Verification items for the finished model (mm, model axes). Face numbers are marked on the shaded views. A direction names the side the tool comes from. Round coordinates to 2 decimals unless told otherwise and drop trailing zeros. Write each loop counter-clockwise with the first axis right and the second up, starting at its lowest first coordinate (ties: lowest second). Pieces come first, ordered by that corner, then holes. Notation, with made-up numbers: (10, 80.5) - (39, 80.5) arc R25 ccw to (39, 92.5) - close; hole circle Ø7 at (-26, 14.25). An arc over 180 degrees is marked (long way). Answer as a JSON object with one key per item and string values. Group by question number.
1) Set-up check for the marked faces 1, 2 and 3: record each of +Z, -Z, +X, -X, +Y, -Y from which the full face is reachable in a straight line by a thin tool's end or side.
2) Section check A-A (y = 0). Enter the section's corners in (x, z).
3) Thickness scan on line 1 (X direction, y = 9.5, z = 255); line 2 (Y direction, x = 18, z = 263.5); line 3 (Z direction, x = -9.5, y = -19.5). Record the ranges inside material, lowest first.
4) Section check D-D (z = 260). Enter the section's corners in (x, y).
5) Section check C-C (x = 19.5). Enter the section's corners in (y, z), then the cut area to 3 significant figures.
6) Mould release check, pull along Y, two halves, no side actions. Record for the marked faces 4, 5 and 6: +Y half, -Y half, draft (parallel to the pull), parting line (faces both ways), or undercut.
7) Go/stop test with flat-tipped pins: pin 1 Ø5 at (x, z) = (2, 259) entering from -Y; pin 2 Ø1.8 at (y, z) = (9.5, 240) entering from +X; pin 3 Ø0.8 at (x, y) = (-1.5, 12.5) entering from -Z; pin 4 Ø5 at (x, y) = (-14.27, 8) entering from -Z. Record where each tip stops, or that it passes through.
8) Section check B-B (z = 252.5). Enter the section's corners in (x, y), then the cut area to 3 significant figures.
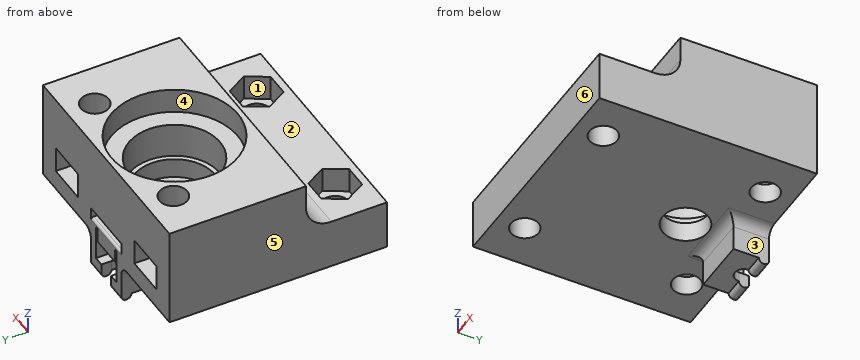
```python
from build123d import *

# Parameters (mm, degrees)
BOSS_EXTRUDE1_DEPTH      = 13.5
BOSS_EXTRUDE2_DEPTH      = 18.5
BOSS_EXTRUDE3_DEPTH      = 5
SKETCH4_W                = 45.922011884
SKETCH4_H                = 20
BOSS_EXTRUDE4_DEPTH      = 13.5
SKETCH2_R                = 4.25
CUT_EXTRUDE1_DEPTH       = 268.629329099
SKETCH6_R                = 9
CUT_EXTRUDE3_DEPTH       = 12
SKETCH7_R                = 12.5
CUT_EXTRUDE4_DEPTH       = 5
BOSS_EXTRUDE5_DEPTH      = 13.5
CUT_EXTRUDE5_REACH       = 210.1
CUT_EXTRUDE5_END_RADIUS  = 45
SKETCH8_R                = 9
CUT_EXTRUDE6_REACH       = 210.1
SKETCH10_R               = 4
SKETCH11_R               = 8
CUT_EXTRUDE7_DEPTH       = 4
SKETCH18_R               = 11
CUT_EXTRUDE9_DEPTH       = 47
CUT_EXTRUDE11_DEPTH      = 268.629329099
CUT_EXTRUDE11_DEPTH_BACK = 268.629329099
SKETCH20_W               = 45.922011884
SKETCH20_H               = 204.425421037
SKETCH21_W               = 45.922011884
SKETCH21_H               = 10
BOSS_EXTRUDE6_DEPTH      = 16
M5_CLEARANCE_HOLE1_D     = 5.5
CUT_EXTRUDE12_DEPTH      = 5
FILLET1_R                = 5
LPATTERN2_COUNT          = 2
LPATTERN2_PITCH          = 32
LPATTERN2_COPY_1_D       = 5.5
CUT_EXTRUDE13_START      = -9.2
SKETCH25_R               = 2.75
CUT_EXTRUDE13_DEPTH      = 5.2
SKETCH26_R               = 8.05
CUT_EXTRUDE14_DEPTH      = 4
SKETCH27_W               = 11
SKETCH27_H               = 7
BOSS_EXTRUDE7_DEPTH      = 5
CUT_EXTRUDE15_DEPTH      = 5
FILLET2_R                = 2
BOSS_EXTRUDE8_DEPTH      = 2
BOSS_EXTRUDE9_DEPTH      = 3.75
SKETCH31_W               = 11
SKETCH31_H               = 2.1
CUT_EXTRUDE16_DEPTH      = 2.5
FILLET3_R                = 0.5
CUT_EXTRUDE17_REACH      = 44.396
SKETCH32_R               = 4.5


with BuildPart() as part:
    # Sketch1 → Boss-Extrude1 (new, symmetric)
    with BuildSketch(Plane(origin=(0, 0, 0), x_dir=(1, 0, 0), z_dir=(0, 1, 0))):
        with BuildLine():
            ThreePointArc((17.220754456, -41.574578963), (0, -45), (-17.220754456, -41.574578963))
            Line((-17.220754456, -41.574578963), (-22.961005942, -55.432771951))
            ThreePointArc((-22.961005942, -55.432771951), (0, -60), (22.961005942, -55.432771951))
            Line((22.961005942, -55.432771951), (17.220754456, -41.574578963))
        make_face()
    extrude(amount=BOSS_EXTRUDE1_DEPTH, both=True)

    # Sketch1_3 → Boss-Extrude2 (add, symmetric)
    with BuildSketch(Plane(origin=(0, 0, 0), x_dir=(1, 0, 0), z_dir=(0, 1, 0))):
        with BuildLine():
            ThreePointArc((19.134171618, -46.193976626), (0, -50), (-19.134171618, -46.193976626))
            Line((-19.134171618, -46.193976626), (-21.04758878, -50.813374288))
            ThreePointArc((-21.04758878, -50.813374288), (0, -55), (21.04758878, -50.813374288))
            Line((21.04758878, -50.813374288), (19.134171618, -46.193976626))
        make_face()
    extrude(amount=BOSS_EXTRUDE2_DEPTH, both=True)

    # Sketch3 → Boss-Extrude3 (add, symmetric)
    with BuildSketch(Plane.XZ):
        with BuildLine():
            Line((-22.961005942, 266), (-22.961005942, 55.432771951))
            ThreePointArc((-22.961005942, 55.432771951), (-20.481139434, 56.39612511), (-17.961005942, 57.248600555))
            Line((-17.961005942, 57.248600555), (-17.961005942, 246))
            Line((-17.961005942, 246), (17.961005942, 246))
            Line((17.961005942, 246), (17.961005942, 57.248600555))
            ThreePointArc((17.961005942, 57.248600555), (20.481139434, 56.39612511), (22.961005942, 55.432771951))
            Line((22.961005942, 55.432771951), (22.961005942, 266))
            Line((22.961005942, 266), (-22.961005942, 266))
        make_face()
    extrude(amount=BOSS_EXTRUDE3_DEPTH, both=True)

    # Sketch4 → Boss-Extrude4 (add, symmetric)
    with BuildSketch(Plane(origin=(0, 0, 0), x_dir=(1, 0, 0), z_dir=(0, 1, 0))):
        with Locations((0, -256)):
            Rectangle(SKETCH4_W, SKETCH4_H)
    extrude(amount=BOSS_EXTRUDE4_DEPTH, both=True)

    # Sketch2 → Cut-Extrude1 (cut, through all)
    with BuildSketch(Plane.XY):
        with Locations(Location((0, 0, 0), (0, 0, 180))):
            Circle(SKETCH2_R)
    extrude(amount=CUT_EXTRUDE1_DEPTH, mode=Mode.SUBTRACT)

    # Sketch6 → Cut-Extrude3 (cut)
    with BuildSketch(Plane.XY.offset(266)):
        Circle(SKETCH6_R)
    extrude(amount=-CUT_EXTRUDE3_DEPTH, mode=Mode.SUBTRACT)

    # Sketch7 → Cut-Extrude4 (cut)
    with BuildSketch(Plane.XY.offset(266)):
        Circle(SKETCH7_R)
    extrude(amount=-CUT_EXTRUDE4_DEPTH, mode=Mode.SUBTRACT)

    # Sketch9 → Boss-Extrude5 (add, symmetric)
    with BuildSketch(Plane(origin=(0, 0, 0), x_dir=(1, 0, 0), z_dir=(0, 1, 0))):
        with BuildLine():
            Line((-22.961005942, -55.432771951), (-22.961005942, -68))
            Line((-22.961005942, -68), (22.961005942, -68))
            Line((22.961005942, -68), (22.961005942, -55.432771951))
            ThreePointArc((22.961005942, -55.432771951), (0, -60), (-22.961005942, -55.432771951))
        make_face()
    extrude(amount=BOSS_EXTRUDE5_DEPTH, both=True)

    # Cut-Extrude5: up to this cylinder (the profile starts outside it)
    cut_extrude5_end = Plane(origin=(0, 0, 0), z_dir=(0, -1, 0)) * Cylinder(CUT_EXTRUDE5_END_RADIUS, 511.2, mode=Mode.PRIVATE)
    # Sketch8 → Cut-Extrude5 (cut, up to the surface)
    with BuildSketch(Plane.XY.offset(60), mode=Mode.PRIVATE) as cut_extrude5_sk1:
        Circle(SKETCH8_R)
    cut_extrude5_tool1 = extrude(cut_extrude5_sk1.sketch, amount=-CUT_EXTRUDE5_REACH, mode=Mode.PRIVATE) - cut_extrude5_end
    add(cut_extrude5_tool1.solids().sort_by_distance((0, 0, 60))[0], mode=Mode.SUBTRACT)

    # Sketch10 → Cut-Extrude6 (cut, up to next)
    with BuildSketch(Plane.XY.offset(60), mode=Mode.PRIVATE) as cut_extrude6_sk1:
        with Locations(Location((0, 0, 0), (0, 0, 180))):
            Circle(SKETCH10_R)
    cut_extrude6_tool1 = extrude(cut_extrude6_sk1.sketch, amount=CUT_EXTRUDE6_REACH, mode=Mode.PRIVATE) & part.part
    add(cut_extrude6_tool1.solids().sort_by_distance((0, 0, 60))[0], mode=Mode.SUBTRACT)

    # Sketch11 → Cut-Extrude7 (cut)
    with BuildSketch(Plane.XY.offset(68)):
        Circle(SKETCH11_R)
    extrude(amount=-CUT_EXTRUDE7_DEPTH, mode=Mode.SUBTRACT)

    # Sketch18 → Cut-Extrude9 (cut)
    with BuildSketch(Plane.XY):
        with Locations(Location((0, 0, 0), (0, 0, 180))):
            Circle(SKETCH18_R)
    extrude(amount=CUT_EXTRUDE9_DEPTH, mode=Mode.SUBTRACT)

    # Sketch20 → Cut-Extrude11 (cut, two sides: drawn at the far end of the back side and taken through both)
    with BuildSketch(Plane(origin=(0, 0, 0), x_dir=(1, 0, 0), z_dir=(0, 1, 0)).offset(-CUT_EXTRUDE11_DEPTH_BACK)):
        with Locations((0, -143.787289482)):
            Rectangle(SKETCH20_W, SKETCH20_H)
    extrude(amount=CUT_EXTRUDE11_DEPTH + CUT_EXTRUDE11_DEPTH_BACK, mode=Mode.SUBTRACT)

    # Sketch21 → Boss-Extrude6 (add)
    with BuildSketch(Plane.XZ.offset(13.5)):
        with Locations((0, 251)):
            Rectangle(SKETCH21_W, SKETCH21_H)
    extrude(amount=BOSS_EXTRUDE6_DEPTH)

    # M5 Clearance Hole1 (through all)
    with Locations(Plane(origin=(0, 0, 246), x_dir=(-1, 0, 0), z_dir=(0, 0, -1))):
        with Locations((-14.26606865, -24)):
            m5_clearance_hole1 = Hole(M5_CLEARANCE_HOLE1_D / 2)

    # Sketch24 → Cut-Extrude12 (cut)
    with BuildSketch(Plane.XY.offset(256)):
        Polygon((18.94260583, -24), (16.60433724, -19.95), (11.92780006, -19.95), (9.58953147, -24), (11.92780006, -28.05), (16.60433724, -28.05), align=None)
    cut_extrude12 = extrude(amount=-CUT_EXTRUDE12_DEPTH, mode=Mode.SUBTRACT)

    # Mirror1: M5 Clearance Hole1 across plane
    add(m5_clearance_hole1.mirror(Plane(origin=(0, 0, 0), x_dir=(0, 0, 1), z_dir=(1, 0, 0))), mode=Mode.SUBTRACT)

    # Mirror2: Cut-Extrude12 across plane
    add(cut_extrude12.mirror(Plane(origin=(0, 0, 0), x_dir=(0, 0, 1), z_dir=(1, 0, 0))), mode=Mode.SUBTRACT)

    # Fillet1
    fillet1_edges = [part.edges().sort_by_distance(p)[0] for p in [
        (0, -13.5, 256),
    ]]
    fillet(fillet1_edges, radius=FILLET1_R)

    # LPattern2: M5 Clearance Hole1 ×2
    with Locations(*[(0, i * LPATTERN2_PITCH, 0) for i in range(1, LPATTERN2_COUNT)]):
        add(m5_clearance_hole1, mode=Mode.SUBTRACT)

    # LPattern2 copy 1 (through all)
    with Locations(Plane(origin=(0, 32, 246), x_dir=(1, 0, 0), z_dir=(0, 0, -1))):
        with Locations((-14.26606865, 24)):
            Hole(LPATTERN2_COPY_1_D / 2)

    # Sketch25 → Cut-Extrude13 (cut)
    # profile 1 of 2: a face of its own
    with BuildSketch(Plane(origin=(0, 0, 246), x_dir=(-1, 0, 0), z_dir=(0, 0, -1)).offset(CUT_EXTRUDE13_START)):
        Polygon((-18.31606865, 13.5), (-18.31606865, 10.33826859), (-14.26606865, 12.67653718), (-10.21606865, 10.33826859), (-10.21606865, 13.5), align=None)
    # profile 2 of 2: a face of its own
    with BuildSketch(Plane(origin=(0, 0, 246), x_dir=(-1, 0, 0), z_dir=(0, 0, -1)).offset(CUT_EXTRUDE13_START)):
        Polygon((-10.21606865, 10.33826859), (-14.26606865, 12.67653718), (-18.31606865, 10.33826859), (-18.31606865, 5.66173141), (-14.26606865, 3.32346282), (-10.21606865, 5.66173141), align=None)
        with Locations((-14.26606865, 8)):
            Circle(SKETCH25_R, mode=Mode.SUBTRACT)
    cut_extrude13 = extrude(amount=CUT_EXTRUDE13_DEPTH, mode=Mode.SUBTRACT)

    # Mirror3: Cut-Extrude13 across plane
    add(cut_extrude13.mirror(Plane(origin=(0, 0, 0), x_dir=(0, 0, 1), z_dir=(1, 0, 0))), mode=Mode.SUBTRACT)

    # Sketch26 → Cut-Extrude14 (cut)
    with BuildSketch(Plane.XY.offset(254)):
        Circle(SKETCH26_R)
    extrude(amount=-CUT_EXTRUDE14_DEPTH, mode=Mode.SUBTRACT)

    # Sketch27 → Boss-Extrude7 (add)
    with BuildSketch(Plane(origin=(0, 0, 246), x_dir=(-1, 0, 0), z_dir=(0, 0, -1))):
        with Locations((0, 10)):
            Rectangle(SKETCH27_W, SKETCH27_H)
    extrude(amount=BOSS_EXTRUDE7_DEPTH)

    # Sketch28 → Cut-Extrude15 (cut)
    with BuildSketch(Plane(origin=(0, 13.5, 0), x_dir=(1, 0, 0), z_dir=(0, 1, 0))):
        Polygon((-3.735, -241), (3.735, -241), (3.735, -248), (3.235, -248), (3.235, -245.2), (-3.235, -245.2), (-3.235, -248), (-3.735, -248), align=None)
    extrude(amount=-CUT_EXTRUDE15_DEPTH, mode=Mode.SUBTRACT)

    # Fillet2
    fillet2_edges = [part.edges().sort_by_distance(p)[0] for p in [
        (5.5, 10, 246),
        (0, 6.5, 246),
        (-5.5, 10, 246),
    ]]
    fillet(fillet2_edges, radius=FILLET2_R)

    # Sketch29 → Boss-Extrude8 (add)
    with BuildSketch(Plane(origin=(0, 0, 241), x_dir=(-1, 0, 0), z_dir=(0, 0, -1))):
        Polygon((5.5, 13.5), (3.735, 13.5), (3.735, 8.5), (-3.735, 8.5), (-3.735, 13.5), (-5.5, 13.5), (-5.5, 6.5), (5.5, 6.5), align=None)
        with BuildLine():
            ThreePointArc((1.75, 11.5), (0, 9.75), (-1.75, 11.5))
            Line((-1.75, 11.5), (-1.75, 13.5))
            Line((-1.75, 13.5), (-3.735, 13.5))
            Line((-3.735, 13.5), (-3.735, 8.5))
            Line((-3.735, 8.5), (3.735, 8.5))
            Line((3.735, 8.5), (3.735, 13.5))
            Line((3.735, 13.5), (1.75, 13.5))
            Line((1.75, 13.5), (1.75, 11.5))
        make_face()
    extrude(amount=BOSS_EXTRUDE8_DEPTH)

    # Sketch30 → Boss-Extrude9 (add)
    with BuildSketch(Plane.ZY.offset(5.5)):
        with BuildLine():
            Line((239, 11.5), (239, 13.5))
            ThreePointArc((239, 13.5), (238, 12.5), (239, 11.5))
        make_face()
    boss_extrude9 = extrude(amount=-BOSS_EXTRUDE9_DEPTH)

    # Mirror4: Boss-Extrude9 across plane
    add(boss_extrude9.mirror(Plane(origin=(0, 0, 0), x_dir=(0, 0, 1), z_dir=(1, 0, 0))))

    # Sketch31 → Cut-Extrude16 (cut)
    with BuildSketch(Plane(origin=(0, 13.5, 0), x_dir=(1, 0, 0), z_dir=(0, 1, 0))):
        with Locations((0, -249.95)):
            Rectangle(SKETCH31_W, SKETCH31_H)
    extrude(amount=-CUT_EXTRUDE16_DEPTH, mode=Mode.SUBTRACT)

    # Fillet3
    fillet3_edges = [part.edges().sort_by_distance(p)[0] for p in [
        (0, 13.5, 248.9),
    ]]
    fillet(fillet3_edges, radius=FILLET3_R)

    # Sketch32 → Cut-Extrude17 (cut, up to next)
    with BuildSketch(Plane(origin=(0, 0, 246), x_dir=(-1, 0, 0), z_dir=(0, 0, -1)), mode=Mode.PRIVATE) as cut_extrude17_sk1:
        with Locations(Location((0, 0, 0), (0, 0, 90))):
            Circle(SKETCH32_R)
    cut_extrude17_tool1 = extrude(cut_extrude17_sk1.sketch, amount=-CUT_EXTRUDE17_REACH, mode=Mode.PRIVATE) & part.part
    add(cut_extrude17_tool1.solids().sort_by_distance((0, 0, 246))[0], mode=Mode.SUBTRACT)


solid = part.part
```
Returned:
{
 "1": {"face 1": "+Z", "face 2": "+Z, +X, -X, -Y", "face 3": "-Z, +X, +Y, -Y"},
 "2": {"outline": "(-22.96, 246) - (-4.5, 246) - (-4.5, 250) - (-8.05, 250) - (-8.05, 254) - (-9, 254) - (-9, 261) - (-12.5, 261) - (-12.5, 266) - (-22.96, 266) - close; (4.5, 246) - (22.96, 246) - (22.96, 266) - (12.5, 266) - (12.5, 261) - (9, 261) - (9, 254) - (8.05, 254) - (8.05, 250) - (4.5, 250) - close"},
 "3": {"line 1": "-22.96 to -18.32, -10.22 to 10.22, 18.32 to 22.96", "line 2": "-13.5 to 13.5", "line 3": "246 to 256"},
 "4": {"outline": "(-22.96, -13.6) - (22.96, -13.6) - (22.96, 13.5) - (-22.96, 13.5) - close; hole circle Ø5.5 at (-14.27, 8); hole circle Ø18 at (0, 0); hole circle Ø5.5 at (14.27, 8)"},
 "5": {"outline": "(-29.5, 246) - (13.5, 246) - (13.5, 266) - (-13.5, 266) - (-13.5, 261) arc R5 cw to (-18.5, 256) - (-29.5, 256) - close", "area": "705 mm2"},
 "6": {"face 4": "undercut", "face 5": "draft", "face 6": "-Y half"},
 "7": {"pin 1": "y = -16.32", "pin 2": "x = 5.5", "pin 3": "z = 238", "pin 4": "through"},
 "8": {"outline": "(-22.96, -29.5) - (22.96, -29.5) - (22.96, 13.5) - (18.32, 13.5) - (18.32, 5.66) - (14.27, 3.32) - (10.22, 5.66) - (10.22, 13.5) - (-10.22, 13.5) - (-10.22, 5.66) - (-14.27, 3.32) - (-18.32, 5.66) - (-18.32, 13.5) - (-22.96, 13.5) - close; hole (-18.94, -24) - (-16.6, -28.05) - (-11.93, -28.05) - (-9.59, -24) - (-11.93, -19.95) - (-16.6, -19.95) - close; hole circle Ø16.1 at (0, 0); hole (9.59, -24) - (11.93, -28.05) - (16.6, -28.05) - (18.94, -24) - (16.6, -19.95) - (11.93, -19.95) - close", "area": "1,510 mm2"}
}
